Work out the finished part from the listing and answer in its coordinate system (mm). Face numbers are marked on the shaded views. A direction names the side the tool comes from. Round coordinates to 2 decimals unless told otherwise and drop trailing zeros. Loops run counter-clockwise (first coordinate to the right, second up) from the corner with the lowest first, then second, coordinate; pieces in that order, holes last. Notation, with made-up numbers: (-38, -5) - (-23, -5) arc R20 cw to (-23, 4) - close; hole circle Ø1 at (2, 34.5). An arc over 180 degrees is marked (long way). Answer as CSV lines item,"result". Start each with the question number.
Q1. The mould has two halves that part along Z. Classify the marked faces 5, 6 and 7: +Z half, -Z half, draft (parallel to the pull), parting line (faces both ways), or undercut.
Q2. Section B-B on y = 31.5 is taken. Write down the section's boundary in (x, z).
Q3. Section D-D on x = -6 is taken. Write down the section's boundary in (y, z), then the cut area to 3 significant figures.
Q4. Each of these flat-tipped pins is pushed along its axis until it touches: pin 1 Ø3 at (x, z) = (36, -6) entering from +Y; pin 2 Ø3 at (x, z) = (-17.5, 18.25) entering from -Y; pin 3 Ø4 at (x, z) = (9.5, 3.5) entering from +Y; pin 4 Ø1.7 at (x, z) = (18.5, 19) entering from +Y. Where does it stop, or does it pass through?
Q5. For the marked faces 1, 2, 3 and 4, determine the directions among +Z, -Z, +X, -X, +Y, -Y from which every point of the face is accessible in a straight line to the end or side of a thin tool.
Q6. Section A-A on z = -1.5 is taken. Write down the section's boundary in (x, y).
Q7. Section C-C on y = 5 is taken. Count the separate pieces of the cut face and the enclosed holes in it, then the cut area to 3 significant figures.
Q8. Straight lines are drawn through the part: L1, parallel to Z at x = 3.5, y = 6; L2, parallel to X at y = 15.8, z = 7.95; L3, parallel to X at y = 3, z = 18.25. For each, find the intervals that lie inside material, in ascending order. Write a range as [from, to].
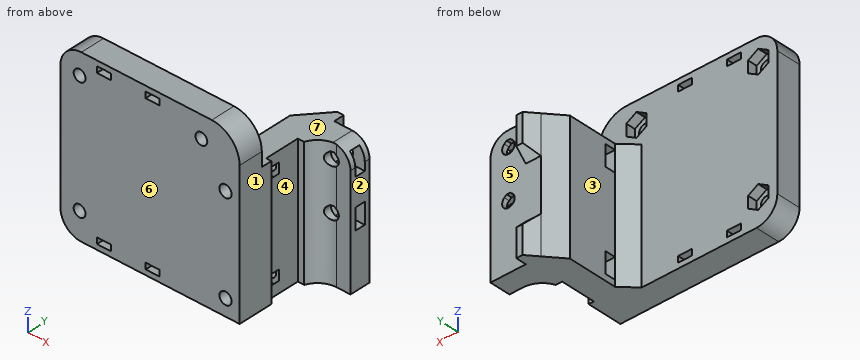
```python
from build123d import *

# Parameters (mm, degrees)
CROQUIS16_W                  = 51.5
CROQUIS16_H                  = 49
SALIENTE_EXTRUIR3_DEPTH      = 7
SALIENTE_EXTRUIR4_DEPTH      = 37
TALADRO_DE_MARGEN_PARA_M31_D = 3.4
REDONDEO1_R                  = 6
REDONDEO2_R                  = 8
CORTAR_EXTRUIR14_DEPTH       = 2.7
REDONDEO3_R                  = 6
CORTAR_EXTRUIR12_DEPTH       = 55.612269684
REDONDEO11_R                 = 5
SALIENTE_EXTRUIR5_DEPTH      = 37
CHAFL_N3_SIZE                = 4
CHAFL_N3_SIZE2               = 4.76701437
CROQUIS29_R                  = 1.75
CORTAR_EXTRUIR17_DEPTH       = 18
CORTAR_EXTRUIR18_DEPTH       = 3
CORTAR_EXTRUIR20_DEPTH       = 3
CORTAR_EXTRUIR21_REACH       = 53.103
CROQUIS31_W                  = 4
CROQUIS31_H                  = 1.75
SALIENTE_EXTRUIR10_DEPTH     = 8
CHAFL_N7_SIZE                = 3
CORTAR_EXTRUIR22_START       = -40
CORTAR_EXTRUIR22_DEPTH       = 40


with BuildPart() as part:
    # Croquis16 → Saliente-Extruir3 (new body)
    with BuildSketch(Plane(origin=(0, 0, 0), x_dir=(1, 0, 0), z_dir=(0, 1, 0))):
        with Locations((2.75, 0)):
            Rectangle(CROQUIS16_W, CROQUIS16_H)
    extrude(amount=SALIENTE_EXTRUIR3_DEPTH)

    # Croquis17 → Saliente-Extruir4 (add)
    with BuildSketch(Plane.XY.offset(-24.5)):
        Polygon((38.5, 30), (38.5, 24), (28.5, 24), (28.5, 7), (20, 7), (20, 30), align=None)
    extrude(amount=SALIENTE_EXTRUIR4_DEPTH)

    # Taladro de margen para M31 (through all)
    with Locations(Plane(origin=(0, 7, 0), x_dir=(1, 0, 0), z_dir=(0, 1, 0))):
        with Locations((-17.5, 16.75), (17.5, -18.25), (-17.5, -18.25)):
            Hole(TALADRO_DE_MARGEN_PARA_M31_D / 2)

    # Redondeo1
    redondeo1_edges = [part.edges().sort_by_distance(p)[0] for p in [
        (-23, 3.5, -24.5),
        (-23, 3.5, 24.5),
    ]]
    fillet(redondeo1_edges, radius=REDONDEO1_R)

    # Redondeo2
    redondeo2_edges = [part.edges().sort_by_distance(p)[0] for p in [
        (28.5, 3.5, 24.5),
    ]]
    fillet(redondeo2_edges, radius=REDONDEO2_R)

    # Croquis24 → Cortar-Extruir14 (cut)
    with BuildSketch(Plane(origin=(0, 7, 0), x_dir=(1, 0, 0), z_dir=(0, 1, 0))):
        Polygon((-17.5, -21.598631561), (-14.6, -19.924315781), (-14.6, -16.575684219), (-17.5, -14.901368439), (-20.4, -16.575684219), (-20.4, -19.924315781), align=None)
        Polygon((17.5, -21.598631561), (20.4, -19.924315781), (20.4, -16.575684219), (17.5, -14.901368439), (14.6, -16.575684219), (14.6, -19.924315781), align=None)
        Polygon((-17.5, 20.098631561), (-20.4, 18.424315781), (-20.4, 15.075684219), (-17.5, 13.401368439), (-14.6, 15.075684219), (-14.6, 18.424315781), align=None)
    extrude(amount=-CORTAR_EXTRUIR14_DEPTH, mode=Mode.SUBTRACT)

    # Redondeo3
    redondeo3_edges = [part.edges().sort_by_distance(p)[0] for p in [
        (28.5, 24, -6),
    ]]
    fillet(redondeo3_edges, radius=REDONDEO3_R)

    # Croquis21 → Cortar-Extruir12 (cut, through all)
    with BuildSketch(Plane(origin=(0, 30, 0), x_dir=(1, 0, 0), z_dir=(0, 1, 0))):
        with BuildLine():
            Line((34.507017697, 4.421120002), (33.85, 3.869816695))
            Line((33.85, 3.869816695), (32.85, 3.869816695))
            Line((32.85, 3.869816695), (32.192982303, 4.421120002))
            ThreePointArc((32.192982303, 4.421120002), (33.35, 7.6), (34.507017697, 4.421120002))
        make_face()
        with BuildLine():
            Line((33.85, -10.035183305), (32.85, -10.035183305))
            Line((32.85, -10.035183305), (32.192982303, -9.483879998))
            ThreePointArc((32.192982303, -9.483879998), (33.35, -6.305), (34.507017697, -9.483879998))
            Line((34.507017697, -9.483879998), (33.85, -10.035183305))
        make_face()
    extrude(amount=-CORTAR_EXTRUIR12_DEPTH, mode=Mode.SUBTRACT)

    # Redondeo11
    redondeo11_edges = [part.edges().sort_by_distance(p)[0] for p in [
        (38.5, 27, 12.5),
    ]]
    fillet(redondeo11_edges, radius=REDONDEO11_R)

    # Croquis26 → Saliente-Extruir5 (add)
    with BuildSketch(Plane(origin=(0, 0, -24.5), x_dir=(-1, 0, 0), z_dir=(0, 0, -1))):
        Polygon((-20, 11), (-16, 7), (-20, 7), align=None)
    extrude(amount=-SALIENTE_EXTRUIR5_DEPTH)

    # Chaflán3
    chafl_n3_edges = [part.edges().sort_by_distance(p)[0] for p in [
        (20, 30, -6),
    ]]
    chafl_n3_side = [part.faces().sort_by_distance(p)[0] for p in [
        (29.053844861, 30, -6.369586264),
    ]]
    chamfer(chafl_n3_edges, length=CHAFL_N3_SIZE, length2=CHAFL_N3_SIZE2, reference=chafl_n3_side[0])

    # Croquis29 → Cortar-Extruir17 (cut)
    with BuildSketch(Plane.XZ):
        with Locations(Location((24.45, -19.75, 0), (0, 0, 270))):
            Circle(CROQUIS29_R)
        with Locations(Location((24.45, 7.95, 0), (0, 0, 270))):
            Circle(CROQUIS29_R)
    extrude(amount=-CORTAR_EXTRUIR17_DEPTH, mode=Mode.SUBTRACT)

    # Croquis30 → Cortar-Extruir18 (cut)
    with BuildSketch(Plane(origin=(0, 11, 0), x_dir=(-1, 0, 0), z_dir=(0, -1, 0))):
        Polygon((-22.746816706, 16.8), (-20, 16.8), (-20, 22.7), (-22.746816706, 22.7), (-26.153183294, 22.7), (-27.856366588, 19.75), (-26.153183294, 16.8), align=None)
        Polygon((-20, -10.9), (-22.746816706, -10.9), (-26.153183294, -10.9), (-27.856366588, -7.95), (-26.153183294, -5), (-22.746816706, -5), (-20, -5), align=None)
    extrude(amount=-CORTAR_EXTRUIR18_DEPTH, mode=Mode.SUBTRACT)

    # Croquis25 → Cortar-Extruir20 (cut)
    with BuildSketch(Plane.XZ.offset(-28.5)):
        Polygon((35.082050808, -2.8), (38.5, -2.8), (38.5, -8.8), (35.082050808, -8.8), (31.617949192, -8.8), (29.885898385, -5.8), (31.617949192, -2.8), align=None)
        Polygon((31.617949192, 11.105), (29.885898385, 8.105), (31.617949192, 5.105), (35.082050808, 5.105), (40.5, 5.105), (40.5, 11.105), (35.082050808, 11.105), align=None)
    extrude(amount=CORTAR_EXTRUIR20_DEPTH, mode=Mode.SUBTRACT)

    # Croquis31 → Cortar-Extruir21 (cut, up to next)
    with BuildSketch(Plane(origin=(0, 7, 0), x_dir=(1, 0, 0), z_dir=(0, 1, 0)), mode=Mode.PRIVATE) as cortar_extruir21_sk1:
        with Locations((3.5, 22.125)):
            Rectangle(CROQUIS31_W, CROQUIS31_H)
    cortar_extruir21_tool1 = extrude(cortar_extruir21_sk1.sketch, amount=-CORTAR_EXTRUIR21_REACH, mode=Mode.PRIVATE) & part.part
    # Croquis31 → Cortar-Extruir21 (cut, up to next)
    with BuildSketch(Plane(origin=(0, 7, 0), x_dir=(1, 0, 0), z_dir=(0, 1, 0)), mode=Mode.PRIVATE) as cortar_extruir21_sk2:
        with Locations((3.5, -22.125)):
            Rectangle(CROQUIS31_W, CROQUIS31_H)
    cortar_extruir21_tool2 = extrude(cortar_extruir21_sk2.sketch, amount=-CORTAR_EXTRUIR21_REACH, mode=Mode.PRIVATE) & part.part
    cortar_extruir21_1 = cortar_extruir21_tool1.solids().sort_by_distance((3.5, 7, -22.125))[0]
    add(cortar_extruir21_1, mode=Mode.SUBTRACT)
    cortar_extruir21_2 = cortar_extruir21_tool2.solids().sort_by_distance((3.5, 7, 22.125))[0]
    add(cortar_extruir21_2, mode=Mode.SUBTRACT)
    cortar_extruir21 = cortar_extruir21_1 + cortar_extruir21_2  # Cortar-Extruir21 as one shape, for the pattern or mirror that repeats it

    # Croquis38 → Saliente-Extruir10 (add)
    with BuildSketch(Plane(origin=(0, 0, -24.5), x_dir=(-1, 0, 0), z_dir=(0, 0, -1))):
        Polygon((-24, 30), (-28.35, 30), (-28.35, 33), (-26.517298894, 33), align=None)
    saliente_extruir10 = extrude(amount=-SALIENTE_EXTRUIR10_DEPTH)

    # Simetría3: Saliente-Extruir10 across plane
    add(saliente_extruir10.mirror(Plane(origin=(0, 0, -6), x_dir=(1, 0, 0), z_dir=(0, 0, -1))))

    # Chaflán7
    chafl_n7_edges = [part.edges().sort_by_distance(p)[0] for p in [
        (26.175, 30, 4.5),
        (26.175, 30, -16.5),
    ]]
    chamfer(chafl_n7_edges, length=CHAFL_N7_SIZE - 0.0001)  # a hair under: the kernel refuses the full size

    # Simetría4: Cortar-Extruir21 across plane
    add(cortar_extruir21.mirror(Plane(origin=(-3.5, 0, 0), x_dir=(0, 0, 1), z_dir=(1, 0, 0))), mode=Mode.SUBTRACT)

    # Croquis39 → Cortar-Extruir22 (cut)
    with BuildSketch(Plane(origin=(0, 0, -24.5), x_dir=(-1, 0, 0), z_dir=(0, 0, -1)).offset(CORTAR_EXTRUIR22_START)):
        with BuildLine():
            Line((-28.5, 10), (-28.5, 18))
            ThreePointArc((-28.5, 18), (-28.586408642, 19.014611872), (-28.843145751, 20))
            Line((-28.843145751, 20), (-30, 20))
            Line((-30, 20), (-30, 10))
            Line((-30, 10), (-28.5, 10))
        make_face()
        Polygon((-27, 20), (-28.5, 20), (-28.5, 18), (-28.5, 10), (-27, 10), align=None)
        with BuildLine():
            Line((-28.5, 18), (-28.5, 20))
            Line((-28.5, 20), (-28.843145751, 20))
            ThreePointArc((-28.843145751, 20), (-28.586408642, 19.014611872), (-28.5, 18))
        make_face()
    extrude(amount=CORTAR_EXTRUIR22_DEPTH, mode=Mode.SUBTRACT)


solid = part.part
```
Findings:
1,face 5,"undercut"
1,face 6,"draft"
1,face 7,"+Z half"
2,outline,"(25.26, -24.5) - (28.35, -24.5) - (28.35, -15) - (25.26, -15) - close; (25.26, 3) - (28.35, 3) - (28.35, 12.5) - (25.26, 12.5) - close"
3,outline,"(0, -24.5) - (7, -24.5) - (7, 24.5) - (0, 24.5) - close"
3,area,"343 mm^2"
4,pin 1,"stops at y = 30"
4,pin 2,"passes through"
4,pin 3,"stops at y = 7"
4,pin 4,"stops at y = 4.3"
5,face 1,"+Z, -Z, +X, -Y"
5,face 2,"+Z, -Z, +X, +Y, -Y"
5,face 3,"+Z, -Z, -X, +Y"
5,face 4,"+Z, -Z, +X"
6,outline,"(-23, 0) - (28.5, 0) - (28.5, 10) - (27, 10) - (27, 20) - (28.84, 20) arc R6 cw to (34.5, 24) - (38.5, 24) - (38.5, 30) - (24, 30) - (20, 25.23) - (20, 11) - (16, 7) - (-23, 7) - close"
7,separate pieces,"1"
7,enclosed holes,"9"
7,area,"2,360 mm^2"
8,L1,"z = [-24.5, -23], [-21.25, 21.25], [23, 24.5]"
8,L2,"x = [20, 22.7], [26.2, 27]"
8,L3,"x = [-23, -19.2], [-15.8, 15.8], [19.2, 28.31]"
